Build history of the part. All positions in model axes, mm. A direction names the side the tool comes from. Coordinates: 2 decimals unless noted, no trailing zeros. Order: outer loops, then holes, each group sorted by start corner. A loop starts at its lowest first (then second) coordinate and runs counter-clockwise, first axis right, second up. Notation, with made-up numbers: M -11.5,38 L 30.5,38 A19 ccw 30.5,50 Z; hole C -27.75,38.25 d10. An arc over 180 degrees is marked long. Write item = value, one per line. Start each with the question number.
Q1. Pin check, flat tips, straight feed: P1, Ø0.6, axis at x = -1.5, z = 0.5, coming from the -Y side; P2, Ø3.5, axis at x = 2, y = -2, coming from the +Z side; P3, Ø6, axis at y = -6, z = 4.5, coming from the +X side. Stop position of each tip, or through.
Q2. Band-saw the part on A-A on y = 3.75. State how many separate pieces and enclosed holes the cut face has, plus the area to 3 significant figures.
Q3. Pull direction X, two halves, no side cores. Call faces 4 (the face through (-9.315, -1.578, 5.059)), 5 (the face through (-13.95, 0.49, -0.46)), 6 (the face through (6.67, 3.61, 3.71)): released by +X, released by -X, zero draft, split by the parting line, or undercut.
Q4. Band-saw the part on B-B on y = -0.5. Write the cut outline in (x, z).
Q5. Drill centre lines: probe 1 along X at (y, z) = (1.75, -1.42); probe 2 along Z at (x, y) = (5.54, 3); probe 3 along X at (y, z) = (2.25, 1.42) (3 decimals). Where is each one in solid material? Low to high.
Q6. 3-axis set-ups, long thin cutter, end or side, ignore diameter. For faces 1 (the face through (-1.399, -7.001, 1.476)), 2 (the face through (2.34, 3.35, 1.12)), 3 (the face through (8.02, -4.59, 3.86)): which of +Z, -Z, +X, -X, +Y, -Y reach the whole face in a straight line?
Autodesk Inventor part; units mm, degrees
ref_plane "YZ Plane" through (0, 0, 0) normal (1, 0, 0) x (0, 1, 0)
ref_plane "XZ Plane" through (0, 0, 0) normal (0, 1, 0) x (-1, 0, 0)
ref_plane "XY Plane" through (0, 0, 0) normal (0, 0, 1) x (1, 0, 0)
sketch "Sketch1" plane through (0, 0, 0) normal (0, 1, 0) x (-1, 0, 0)
  line L0 (-14.405, 6.275) -> (14.405, 6.275)
  line L1 (15.405, 5.275) -> (15.405, -5.275)
  line L2 (14.405, -6.275) -> (-14.405, -6.275)
  line L3 (-15.405, -5.275) -> (-15.405, 5.275)
  arc A0 (-14.405, 6.275) -> (-15.405, 5.275) centre (-14.405, 5.275) ccw
  arc A1 (15.405, 5.275) -> (14.405, 6.275) centre (14.405, 5.275) ccw
  arc A2 (14.405, -6.275) -> (15.405, -5.275) centre (14.405, -5.275) ccw
  arc A3 (-15.405, -5.275) -> (-14.405, -6.275) centre (-14.405, -5.275) ccw
  circle A4 centre (12.495, 0) radius 1.525
  circle A5 centre (-12.495, 0) radius 1.525
  point P0 (0, 0)
  point P1 (-15.405, 6.275)
  point P2 (15.405, -6.275)
  point P3 (15.405, 6.275)
  dimension "d0" = 30.81
  dimension "d1" = 12.55
  dimension "d2" = 6.275
  dimension "d3" = 15.405
  dimension "d4" = 1
  dimension "d16" = 3.05
  dimension "d17" = 3.05
  dimension "d18" = 24.99
  dimension "d19" = 12.495
extrude "Extrusion1" add sketch "Sketch1" along normal blind 1
sketch "Sketch2" plane through (0, 1, 0) normal (0, 1, 0) x (1, 0, 0)
  line L0 (-7.0582, 3.95) -> (7.0582, 3.95)
  line L1 (8.25, 3.95) -> (8.25, -3.95)
  line L2 (6.0179, -3.95) -> (-6.0179, -3.95)
  line L3 (-8.25, -3.95) -> (-8.25, 3.95)
  line L4 (-8.0431, 2.7764) -> (-7.0027, -3.1236)
  line L5 (8.0431, 2.7764) -> (7.0027, -3.1236)
  arc A0 (-7.0582, 3.95) -> (-8.0431, 2.7764) centre (-7.0582, 2.95) ccw
  arc A1 (-7.0027, -3.1236) -> (-6.0179, -3.95) centre (-6.0179, -2.95) ccw
  arc A2 (6.0179, -3.95) -> (7.0027, -3.1236) centre (6.0179, -2.95) ccw
  arc A3 (8.0431, 2.7764) -> (7.0582, 3.95) centre (7.0582, 2.95) ccw
  point P0 (0, 0)
  dimension "d7" = 16.5
  dimension "d8" = 7.9
  dimension "d9" = 3.95
  dimension "d10" = 8.25
  dimension "d11" = 10
  dimension "d12" = 10
  dimension "d13" = 1
extrude "Extrusion2" add sketch "Sketch2" along normal blind 5.8
sketch "Sketch3" plane through (0, 0, 0) normal (0, -1, 0) x (1, 0, 0)
  line L0 (-8.6, 5.36) -> (8.6, 5.36)
  line L1 (9.6, 4.36) -> (9.6, -4.36)
  line L2 (8.6, -5.36) -> (-8.6, -5.36)
  line L3 (-9.6, -4.36) -> (-9.6, 4.36)
  arc A0 (-8.6, 5.36) -> (-9.6, 4.36) centre (-8.6, 4.36) ccw
  arc A1 (9.6, 4.36) -> (8.6, 5.36) centre (8.6, 4.36) ccw
  arc A2 (8.6, -5.36) -> (9.6, -4.36) centre (8.6, -4.36) ccw
  arc A3 (-9.6, -4.36) -> (-8.6, -5.36) centre (-8.6, -4.36) ccw
  point P0 (0, 0)
  point P1 (-9.6, 5.36)
  point P2 (9.6, -5.36)
  point P3 (9.6, 5.36)
  dimension "d20" = 19.2
  dimension "d21" = 10.72
  dimension "d22" = 5.36
  dimension "d23" = 9.6
  dimension "d24" = 1
extrude "Extrusion3" add sketch "Sketch3" along normal blind 4.1
fillet "Fillet1" radius 0.9 8 edges at (9.3071, -4.1, -5.0671) (9.6, -4.1, 0) (9.3071, -4.1, 5.0671) (0, -4.1, 5.36) (-9.3071, -4.1, 5.0671) (-9.6, -4.1, 0) (-9.3071, -4.1, -5.0671) (0, -4.1, -5.36)
sketch "Sketch4" plane through (0, -4.1, 0) normal (0, -1, 0) x (1, 0, 0)
  line L0 (-7.2476, 4.1431) -> (7.3248, 4.1431)
  line L1 (8.3248, 3.1431) -> (8.3248, -3.1174)
  line L2 (7.3248, -4.1174) -> (-7.2476, -4.1174)
  line L3 (-8.2476, -3.1174) -> (-8.2476, 3.1431)
  arc A0 (-7.2476, 4.1431) -> (-8.2476, 3.1431) centre (-7.2476, 3.1431) ccw
  arc A1 (8.3248, 3.1431) -> (7.3248, 4.1431) centre (7.3248, 3.1431) ccw
  arc A2 (7.3248, -4.1174) -> (8.3248, -3.1174) centre (7.3248, -3.1174) ccw
  arc A3 (-8.2476, -3.1174) -> (-7.2476, -4.1174) centre (-7.2476, -3.1174) ccw
  point P0 (0, 0)
  point P1 (-8.2476, 4.1431)
  point P2 (8.3248, -4.1174)
  point P3 (8.3248, 4.1431)
  point P4 (-8.2476, -4.1174)
  dimension "d30" = 1
extrude "Extrusion4" add sketch "Sketch4" along normal blind 1
sketch "Sketch5" plane through (0, 1, 0) normal (0, 1, 0) x (1, 0, 0)
  line L0 (7.3082, 4.0255) -> (-7.3082, 4.0255)
  circle A0 centre (-5.54, 1.42) radius 1
  circle A1 centre (-4.155, -1.42) radius 1
  circle A2 centre (-2.77, 1.42) radius 1
  circle A3 centre (0, 1.42) radius 1
  circle A4 centre (2.77, 1.42) radius 1
  circle A5 centre (5.54, 1.42) radius 1
  circle A6 centre (-1.385, -1.42) radius 1
  circle A7 centre (1.385, -1.42) radius 1
  circle A8 centre (4.155, -1.42) radius 1
  point P0 (0, 0)
  dimension "d31" = 5.54
  dimension "d32" = 4.155
  dimension "d34" = 1.42
  dimension "d35" = 1.42
  dimension "d36" = 2
  dimension "d37" = 2
  dimension "d40" = 2.77
  dimension "d47" = 2.77
extrude "Extrusion5" add sketch "Sketch5" along normal blind 7.35 and the other way blind 9.4
sketch "Sketch6" plane through (-9.6, 0, -4.36) normal (-1, 0, 0) x (0, 0, 1)
  line L0 (0, 0) -> (0, -3.2)
  line L1 (1.538, -5.6397) -> (2.3945, -5.6397)
  line L2 (2.3945, -5.6397) -> (3.6462, -8.7799)
  line L3 (3.6462, -8.7799) -> (1.538, -8.7799)
  line L4 (1.538, -8.7799) -> (1.538, -5.6397)
  line L5 (4.4367, -5.6397) -> (5.2932, -5.6397)
  line L6 (5.2932, -5.6397) -> (6.5449, -8.7799)
  line L7 (6.5449, -8.7799) -> (4.4367, -8.7799)
  line L8 (4.4367, -8.7799) -> (4.4367, -5.6397)
  point P0 (4.36, 0)
extrude "Extrusion6" cut sketch "Sketch6" against normal through all
fillet "Fillet2" radius 0.5 8 edges at (6.6607, 6.8, 3.716) (7.5229, 6.8, 0.1736) (7.8243, 6.8, -3.5928) (0, 6.8, -3.95) (-7.8243, 6.8, -3.5928) (-7.5229, 6.8, 0.1736) (-6.6607, 6.8, 3.716) (0, 6.8, 3.95)
sketch "Sketch7" plane through (0, 6.8, 0) normal (0, 1, 0) x (1, 0, 0)
  circle A0 centre (4.155, -1.42) radius 1
  circle A1 centre (-1.385, -1.42) radius 1
  circle A2 centre (2.77, 1.42) radius 1
  circle A3 centre (-2.77, 1.42) radius 1
  circle A4 centre (-5.54, 1.42) radius 1
  circle A5 centre (-4.155, -1.42) radius 1
  circle A6 centre (0, 1.42) radius 1
  circle A7 centre (5.54, 1.42) radius 1
  circle A8 centre (1.385, -1.42) radius 1
  line L0 (-7.0582, 3.45) -> (7.0582, 3.45)
  circle A9 centre (-5.54, 1.42) radius 1.05
  circle A10 centre (-4.155, -1.42) radius 1.05
  circle A11 centre (-2.77, 1.42) radius 1.05
  circle A12 centre (0, 1.42) radius 1.05
  circle A13 centre (2.77, 1.42) radius 1.05
  circle A14 centre (5.54, 1.42) radius 1.05
  circle A15 centre (-1.385, -1.42) radius 1.05
  circle A16 centre (1.385, -1.42) radius 1.05
  circle A17 centre (4.155, -1.42) radius 1.05
  point P0 (0, 0)
  dimension "d59" = 2.1
  dimension "d60" = 2.1
  dimension "d63" = 2.77
  dimension "d70" = 2.77
extrude "Extrusion7" cut sketch "Sketch7" along normal mid plane 14 contours A0 | A1 | A2 | A3 | A4 | A5 | A6 | A7 | A8
properties part number "DSUB_9_Female"
Recorded:
q1.P1 = -5.64
q1.P2 = 5.36
q1.P3 = 9.6
q2.separate_pieces = 1
q2.enclosed_holes = 9
q2.area = 90.2 mm2
q3.face_4 = released by -X
q3.face_5 = undercut
q3.face_6 = released by +X
q4.outline = M -9.6,-4.36 A1 ccw -8.6,-5.36 L 8.6,-5.36 A1 ccw 9.6,-4.36 L 9.6,4.36 A1 ccw 8.6,5.36 L -8.6,5.36 A1 ccw -9.6,4.36 Z
q5.probe_1 = -7.8 to -6.54, -4.54 to -3.77, -1.77 to -1, 1 to 1.77, 3.77 to 4.54, 6.54 to 7.8
q5.probe_2 = -3.95 to -2.42, -0.42 to 3.95
q5.probe_3 = -7.303 to -5.155, -3.155 to -2.385, -0.385 to 0.385, 2.385 to 3.155, 5.155 to 7.303
q6.face_1 = +X, -X, -Y
q6.face_2 = +Y
q6.face_3 = +Z, +X, -Y
